Read the model definition and answer for the solid it produces. Units are mm, in the model's axes. Face numbers are marked on the shaded views. A direction names the side the tool comes from. Give positions to 0.01 mm unless a question says otherwise; leave off trailing zeros. Loops run counter-clockwise (first coordinate to the right, second up) from the corner with the lowest first, then second, coordinate; pieces in that order, holes last. Notation, with made-up numbers: (58.5, 74) - (84.5, 74) arc R22 ccw to (84.5, 82) - close; hole circle Ø11 at (6, -2.5). An arc over 180 degrees is marked (long way). Use a Markdown table: item, result. Add a question column.
Item 1: A cutting plane is placed at A-A (z = 4.25). Give the number of separate pieces and of enclosed holes in the cut face, plus the area to 4 significant figures.
Item 2: A cutting plane is placed at B-B (x = -1.1). Determine the outline of the cut face in (y, z) (3 decimals).
Item 3: Consider probe 1 along Y at (x, z) = (0, 7.25); probe 2 along Y at (x, z) = (0.9, 1) (3 decimals); probe 3 along Z at (x, y) = (-0.6, 5.25). Determine where each line is inside the solid, lowest interval first. Write a range as [from, to].
Item 4: A cutting plane is placed at C-C (z = 0.5). Determine the outline of the cut face in (x, y) (3 decimals).
Item 5: Each of these flat-tipped pins is pushed along its axis until it touches: P1, Ø1, axis at x = -1, y = 2.5, coming from the -Z side; P2, Ø0.8, axis at y = 3.5, z = -1, coming from the +X side; P3, Ø0.8, axis at x = 0, z = 5.5, coming from the -Y side. Where does it stop, or does it pass through?
Item 6: A cutting plane is placed at D-D (y = 6.5). Determine the outline of the cut face in (x, z).
Item 7: For a pull along Y with two mould halves and no side action, classify the marked faces 1, 2 and 3 as +Y half, -Y half, draft (parallel to the pull), parting line (faces both ways), or undercut.
Item 8: Which of the six approach directions +Z, -Z, +X, -X, +Y, -Y give full straight-line access (tool end or side, diameter ignored) to the marked faces 4 and 5?
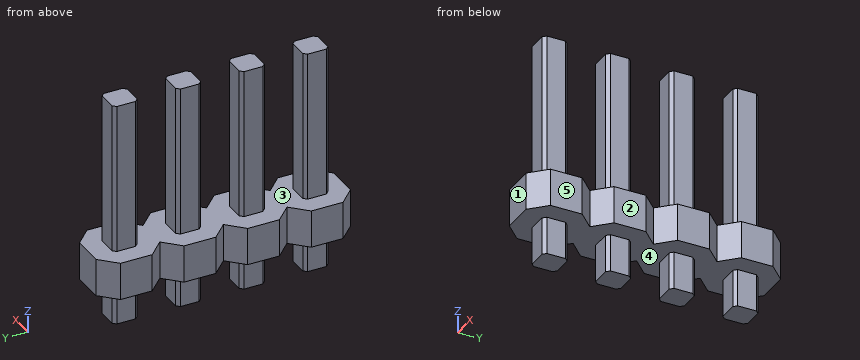
from build123d import *

# Parameters (mm, degrees)
BOSS_EXTRUDE1_DEPTH      = 1.5
BOSS_EXTRUDE2_DEPTH      = 6
BOSS_EXTRUDE2_DEPTH_BACK = 3


with BuildPart() as part:
    # Sketch1 → Boss-Extrude1 (new body)
    with BuildSketch(Plane.XY):
        Polygon((-0.635, 10.16), (0.635, 10.16), (1.27, 9.525), (1.27, 8.255), (0.635, 7.62), (1.27, 6.985), (1.27, 5.715), (0.635, 5.08), (1.27, 4.445), (1.27, 3.175), (0.635, 2.54), (1.27, 1.905), (1.27, 0.635), (0.635, 0), (-0.635, 0), (-1.27, 0.635), (-1.27, 1.905), (-0.635, 2.54), (-1.27, 3.175), (-1.27, 4.445), (-0.635, 5.08), (-1.27, 5.715), (-1.27, 6.985), (-0.635, 7.62), (-1.27, 8.255), (-1.27, 9.525), align=None)
    extrude(amount=BOSS_EXTRUDE1_DEPTH)

    # Sketch2 → Boss-Extrude2 (add, two sides: drawn at the far end of the back side and taken through both)
    with BuildSketch(Plane.XY.offset(1.5).offset(-BOSS_EXTRUDE2_DEPTH_BACK)):
        Polygon((0.5, 9.265), (0.375, 9.39), (-0.375, 9.39), (-0.5, 9.265), (-0.5, 8.515), (-0.375, 8.39), (0.375, 8.39), (0.5, 8.515), align=None)
        Polygon((0.5, 6.725), (0.375, 6.85), (-0.375, 6.85), (-0.5, 6.725), (-0.5, 5.975), (-0.375, 5.85), (0.375, 5.85), (0.5, 5.975), align=None)
        Polygon((0.5, 4.185), (0.375, 4.31), (-0.375, 4.31), (-0.5, 4.185), (-0.5, 3.435), (-0.375, 3.31), (0.375, 3.31), (0.5, 3.435), align=None)
        Polygon((0.5, 1.645), (0.375, 1.77), (-0.375, 1.77), (-0.5, 1.645), (-0.5, 0.895), (-0.375, 0.77), (0.375, 0.77), (0.5, 0.895), align=None)
    extrude(amount=BOSS_EXTRUDE2_DEPTH + BOSS_EXTRUDE2_DEPTH_BACK)


solid = part.part
Geometry says:
| question | item | result |
|---|---|---|
| 1 | separate pieces | 4 |
| 1 | enclosed holes | 0 |
| 1 | area | 3.875 mm² |
| 2 | outline | (0.465, 0) - (2.075, 0) - (2.075, 1.5) - (0.465, 1.5) - close; (3.005, 0) - (4.615, 0) - (4.615, 1.5) - (3.005, 1.5) - close; (5.545, 0) - (7.155, 0) - (7.155, 1.5) - (5.545, 1.5) - close; (8.085, 0) - (9.695, 0) - (9.695, 1.5) - (8.085, 1.5) - close |
| 3 | probe 1 | [0.77, 1.77], [3.31, 4.31], [5.85, 6.85], [8.39, 9.39] |
| 3 | probe 2 | [0.265, 2.275], [2.805, 4.815], [5.345, 7.355], [7.885, 9.895] |
| 3 | probe 3 | [0, 1.5] |
| 4 | outline | (-1.27, 0.635) - (-0.635, 0) - (0.635, 0) - (1.27, 0.635) - (1.27, 1.905) - (0.635, 2.54) - (1.27, 3.175) - (1.27, 4.445) - (0.635, 5.08) - (1.27, 5.715) - (1.27, 6.985) - (0.635, 7.62) - (1.27, 8.255) - (1.27, 9.525) - (0.635, 10.16) - (-0.635, 10.16) - (-1.27, 9.525) - (-1.27, 8.255) - (-0.635, 7.62) - (-1.27, 6.985) - (-1.27, 5.715) - (-0.635, 5.08) - (-1.27, 4.445) - (-1.27, 3.175) - (-0.635, 2.54) - (-1.27, 1.905) - close |
| 5 | P1 | z = 0 |
| 5 | P2 | x = 0.5 |
| 5 | P3 | y = 0.77 |
| 6 | outline | (-1.27, 0) - (-0.5, 0) - (-0.5, -1.5) - (0.5, -1.5) - (0.5, 0) - (1.27, 0) - (1.27, 1.5) - (0.5, 1.5) - (0.5, 7.5) - (-0.5, 7.5) - (-0.5, 1.5) - (-1.27, 1.5) - close |
| 7 | face 1 | -Y half |
| 7 | face 2 | draft |
| 7 | face 3 | undercut |
| 8 | face 4 | -Z |
| 8 | face 5 | +Z, -Z, +X, +Y, -Y |
